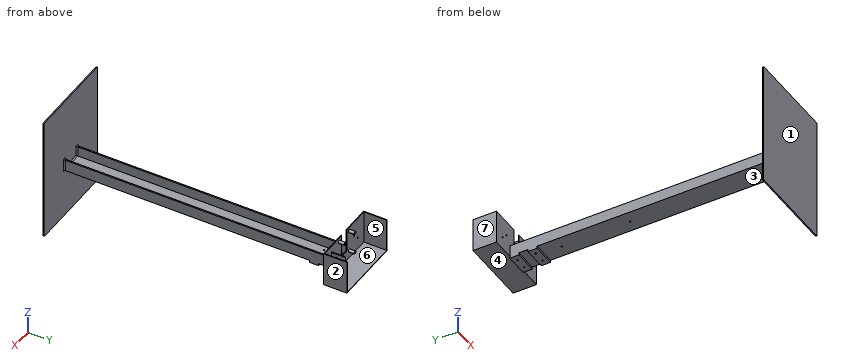
```python
from build123d import *

# Parameters (mm, degrees)
SKETCH1_W             = 400
SKETCH1_H             = 550
BOSS_EXTRUDE2_DEPTH   = 5
EXTRUDE_THIN1_DEPTH   = 1200
FILLET3_R             = 5
BOSS_EXTRUDE4_DEPTH   = 3
SKETCH8_W             = 3
SKETCH8_H             = 70
BOSS_EXTRUDE5_DEPTH   = 60.4
SKETCH9_R             = 15
CUT_EXTRUDE2_DEPTH    = 3
SKETCH10_R            = 1.5
CUT_EXTRUDE3_DEPTH    = 3
SKETCH12_R            = 6.5
BOSS_EXTRUDE6_DEPTH   = 25
SKETCH13_R            = 3
CUT_EXTRUDE5_DEPTH    = 3
EXTRUDE_THIN2_DEPTH   = 100
F_6_0MM_DOWEL_HOLE1_D = 6
SKETCH18_W            = 100
SKETCH18_H            = 40
BOSS_EXTRUDE7_DEPTH   = 10
F_6_0MM_DOWEL_HOLE2_D = 6


with BuildPart() as part:
    # Sketch1 → Boss-Extrude2 (new body)
    with BuildSketch(Plane(origin=(0, 0, 0), x_dir=(1, 0, 0), z_dir=(0, 1, 0))):
        with Locations((200, -275)):
            Rectangle(SKETCH1_W, SKETCH1_H)
    extrude(amount=BOSS_EXTRUDE2_DEPTH)

    # Sketch2 → Extrude-Thin1 (add)
    with BuildSketch(Plane(origin=(0, 5, 0), x_dir=(1, 0, 0), z_dir=(0, 1, 0))):
        Polygon((150, -270), (150, -220), (250, -220), (250, -270), (244, -270), (244, -226), (156, -226), (156, -270), align=None)
    extrude(amount=EXTRUDE_THIN1_DEPTH)

    # Fillet3
    fillet3_edges = [part.edges().sort_by_distance(p)[0] for p in [
        (244, 5, 248),
        (156, 5, 248),
        (200, 5, 226),
        (153, 5, 270),
        (150, 5, 245),
        (200, 5, 220),
        (250, 5, 245),
        (247, 5, 270),
        (0, 2.5, 0),
        (400, 2.5, 0),
        (400, 2.5, 550),
        (0, 2.5, 550),
    ]]
    fillet(fillet3_edges, radius=FILLET3_R)

    # Sketch7 → Boss-Extrude4 (add)
    with BuildSketch(Plane(origin=(0, 1205, 0), x_dir=(1, 0, 0), z_dir=(0, 1, 0))):
        Polygon((350, -220), (50, -220), (50, -370), (181, -370), (181, -267.719735963), (219, -267.719735963), (219, -370), (350, -370), align=None)
    extrude(amount=BOSS_EXTRUDE4_DEPTH)

    # Sketch8 → Boss-Extrude5 (add)
    with BuildSketch(Plane(origin=(0, 1208, 0), x_dir=(1, 0, 0), z_dir=(0, 1, 0))):
        with Locations((293.5, -305)):
            Rectangle(SKETCH8_W, SKETCH8_H)
    extrude(amount=BOSS_EXTRUDE5_DEPTH)

    # Sketch9 → Cut-Extrude2 (cut)
    with BuildSketch(Plane(origin=(295, 0, 0), x_dir=(0, 0, -1), z_dir=(1, 0, 0))):
        with Locations((-306.55, 1238.2)):
            Circle(SKETCH9_R)
    extrude(amount=-CUT_EXTRUDE2_DEPTH, mode=Mode.SUBTRACT)

    # Sketch10 → Cut-Extrude3 (cut)
    with BuildSketch(Plane.ZY.offset(-292)):
        with Locations((306.55, 1258.2)):
            Circle(SKETCH10_R)
        with Locations((289.229491924, 1228.2)):
            Circle(SKETCH10_R)
        with Locations((323.870508076, 1228.2)):
            Circle(SKETCH10_R)
    extrude(amount=-CUT_EXTRUDE3_DEPTH, mode=Mode.SUBTRACT)

    # Sketch12 → Boss-Extrude6 (add)
    with BuildSketch(Plane(origin=(0, 1208, 0), x_dir=(1, 0, 0), z_dir=(0, 1, 0))):
        with Locations(Location((162, -352, 0), (0, 0, 270))):
            Circle(SKETCH12_R)
        with Locations(Location((162, -257, 0), (0, 0, 270))):
            Circle(SKETCH12_R)
        with Locations(Location((238, -257, 0), (0, 0, 270))):
            Circle(SKETCH12_R)
        with Locations(Location((238, -352, 0), (0, 0, 270))):
            Circle(SKETCH12_R)
    extrude(amount=BOSS_EXTRUDE6_DEPTH)

    # Sketch13 → Cut-Extrude5 (cut)
    with BuildSketch(Plane(origin=(0, 1208, 0), x_dir=(1, 0, 0), z_dir=(0, 1, 0))):
        with Locations(Location((126, -304.5, 0), (0, 0, 270))):
            Circle(SKETCH13_R)
        with Locations(Location((98.09349971, -275.842937318, 0), (0, 0, 270))):
            Circle(SKETCH13_R)
    extrude(amount=-CUT_EXTRUDE5_DEPTH, mode=Mode.SUBTRACT)

    # Sketch15 → Extrude-Thin2 (add)
    with BuildSketch(Plane(origin=(0, 1208, 0), x_dir=(1, 0, 0), z_dir=(0, 1, 0))):
        Polygon((350, -370), (350, -220), (50, -220), (50, -370), (53, -370), (53, -223), (347, -223), (347, -370), align=None)
    extrude(amount=EXTRUDE_THIN2_DEPTH)

    # Ø6.0mm Dowel Hole1 (through all)
    with Locations(Plane(origin=(0, 0, 220), x_dir=(-1, 0, 0), z_dir=(0, 0, -1))):
        with Locations((-200, 1005), (-200, 705)):
            Hole(F_6_0MM_DOWEL_HOLE1_D / 2)

    # Sketch18 → Boss-Extrude7 (add)
    with BuildSketch(Plane(origin=(0, 0, 220), x_dir=(-1, 0, 0), z_dir=(0, 0, -1))):
        with Locations((-200, 1185)):
            Rectangle(SKETCH18_W, SKETCH18_H)
        with Locations((-200, 1105)):
            Rectangle(SKETCH18_W, SKETCH18_H)
    extrude(amount=BOSS_EXTRUDE7_DEPTH)

    # Ø6.0mm Dowel Hole2 (through all)
    with Locations(Plane(origin=(0, 0, 210), x_dir=(-1, 0, 0), z_dir=(0, 0, -1))):
        with Locations((-225, 1185), (-175, 1185), (-175, 1105), (-225, 1105)):
            Hole(F_6_0MM_DOWEL_HOLE2_D / 2)


solid = part.part
```
Read the model definition and answer for the solid it produces. Units are mm, in the model's axes. Face numbers are marked on the shaded views. A direction names the side the tool comes from. Coordinates: 2 decimals unless noted, no trailing zeros. Order: outer loops, then holes, each group sorted by start corner. A loop starts at its lowest first (then second) coordinate and runs counter-clockwise, first axis right, second up. Notation, with made-up numbers: (39, 36.5) - (86, 36.5) arc R13 cw to (86, 41.5) - close; hole circle Ø3 at (29.25, -12.75). An arc over 180 degrees is marked (long way). Answer as a JSON object with one key per item and string values. Group by question number.
Item 1: Consider probe 1 along X at (y, z) = (1185, 218); probe 2 along Z at (x, y) = (293, 1258); probe 3 along Y at (x, z) = (225, 216). Determine where each line is inside the solid, lowest interval first. Write a range as from..to.
Item 2: A tool of negligible diameter and unlimited length cuts with its end or side. For the marked faces 1, 2 and 3, from which of +Z, -Z, +X, -X, +Y, -Y can it reach the whole face along a straight path? Write none if from no direction.
Item 3: Section B-B (y = 671) is taken. Give the vertices of the cut face in (x, z), plus the area to 3 significant figures.
Item 4: Section D-D (x = 367.5) is taken. Give the vertices of the cut face in (y, z).
Item 5: The mould has two halves that part along X. Classify the marked faces 4, 5, 6 and 7: +X half, -X half, draft (parallel to the pull), parting line (faces both ways), or undercut.
Item 6: Section C-C (z = 67) is taken. Give the vertices of the cut face in (x, y).
Item 7: Section A-A (x = 65) is taken. Give the vertices of the cut face in (y, z), plus the area to 3 significant figures.
Item 8: Flat-ended cylindrical pins translate along their axes: P1, Ø14.5, axis at x = 236, z = 256.5, coming from the +Y side; P2, Ø8, axis at x = 206.5, z = 214, coming from the +Y side; P3, Ø8, axis at x = 191.5, y = 1036.5, coming from the +Z side. Find the tip coordinate at first contact, or state that the pin passes through.
Results are:
{
 "1": {"probe 1": "x = 150..172, 178..222, 228..250", "probe 2": "z = 220..223, 270..305.06, 308.04..340", "probe 3": "y = 0..5.1, 1085..1102, 1108..1125, 1165..1182, 1188..1205"},
 "2": {"face 1": "+Z, -Z, +X, -X, -Y", "face 2": "+Z, -Z, +X, +Y", "face 3": "-Z, +X, -X"},
 "3": {"outline": "(150, 220) - (250, 220) - (250, 270) - (244, 270) - (244, 226) - (156, 226) - (156, 270) - (150, 270) - close", "area": "1,130 mm^2"},
 "4": {"outline": "(0, 0) - (5, 0) - (5, 550) - (0, 550) - close"},
 "5": {"face 4": "draft", "face 5": "undercut", "face 6": "undercut", "face 7": "-X half"},
 "6": {"outline": "(0, 0) - (400, 0) - (400, 5) - (0, 5) - close"},
 "7": {"outline": "(0, 0) - (5, 0) - (5, 550) - (0, 550) - close; (1205, 220) - (1308, 220) - (1308, 223) - (1208, 223) - (1208, 370) - (1205, 370) - close", "area": "3,500 mm^2"},
 "8": {"P1": "stops at y = 1233", "P2": "stops at y = 1205", "P3": "stops at z = 226"}
}
